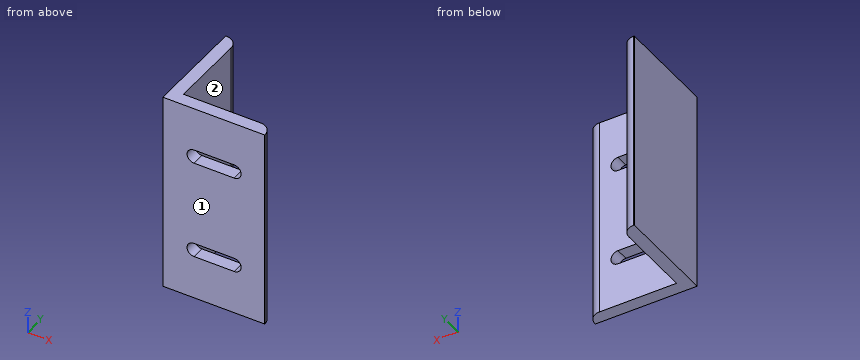
```python
from build123d import *

# Parameters (mm, degrees)
BOSS_EXTRUDE1_DEPTH = 100.4
CUT_EXTRUDE1_DEPTH  = 10


with BuildPart() as part:
    # Sketch1 → Boss-Extrude1 (new body)
    with BuildSketch(Plane.XY):
        with BuildLine():
            Line((44.8, 6.35), (12.35, 6.35))
            Line((12.35, 6.35), (6.35, 6.35))
            Line((6.35, 6.35), (6.35, 44.8))
            ThreePointArc((6.35, 44.8), (4.592640687, 49.042640687), (0.35, 50.8))
            Line((0.35, 50.8), (0, 50.8))
            Line((0, 50.8), (0, 6.35))
            Line((0, 6.35), (0, 0))
            Line((0, 0), (6.35, 0))
            Line((6.35, 0), (50.8, 0))
            Line((50.8, 0), (50.8, 0.35))
            ThreePointArc((50.8, 0.35), (49.042640687, 4.592640687), (44.8, 6.35))
        make_face()
    extrude(amount=BOSS_EXTRUDE1_DEPTH)

    # Sketch2 → Cut-Extrude1 (cut)
    with BuildSketch(Plane(origin=(0, 6.35, 0), x_dir=(1, 0, 0), z_dir=(0, 1, 0))):
        with BuildLine():
            Line((15.575, -21.9), (35.575, -21.9))
            ThreePointArc((35.575, -21.9), (39.075, -25.4), (35.575, -28.9))
            Line((35.575, -28.9), (15.575, -28.9))
            ThreePointArc((15.575, -28.9), (12.075, -25.4), (15.575, -21.9))
        make_face()
        with BuildLine():
            Line((15.575, -78.5), (35.575, -78.5))
            ThreePointArc((35.575, -78.5), (39.075, -75), (35.575, -71.5))
            Line((35.575, -71.5), (15.575, -71.5))
            ThreePointArc((15.575, -71.5), (12.075, -75), (15.575, -78.5))
        make_face()
    extrude(amount=-CUT_EXTRUDE1_DEPTH, mode=Mode.SUBTRACT)


solid = part.part
```
Build history of the part. All positions in model axes, mm. Face numbers are marked on the shaded views. A direction names the side the tool comes from. Round coordinates to 2 decimals unless told otherwise and drop trailing zeros. Write each loop counter-clockwise with the first axis right and the second up, starting at its lowest first coordinate (ties: lowest second). Pieces come first, ordered by that corner, then holes.
1) Pin check, flat tips, straight feed: pin 1 (1 mm diameter, centred on x = 25.5, z = 51, fed in from +Y); pin 2 (19 mm diameter, centred on y = 30.5, z = 72.5, fed in from +X). Stop position of each tip, or through.
2) Band-saw the part on A-A, the plane x = 24.5. List the corners of the cut face in (y, z), and give its area (3 significant figures).
3) Drill centre lines: probe 1 along Z at (x, y) = (37, 3); probe 2 along X at (y, z) = (35.5, 75). Where is each one in solid material? Low to high.
4) Band-saw the part on C-C, the plane z = 55. List the corners of the cut face in (x, y).
5) 3-axis set-ups, long thin cutter, end or side, ignore diameter. For the marked faces 1 and 2: which of +Z, -Z, +X, -X, +Y, -Y reach the whole face in a straight line?
6) Band-saw the part on B-B, the plane z = 75. List the corners of the cut face in (x, y) (3 decimals), and give its area (3 significant figures).
7) Band-saw the part on D-D, the plane y = 15.5. List the corners of the cut face in (x, z).
Ans:
1. pin 1: stops at y = 6.35
1. pin 2: stops at x = 6.35
2. outline: (0, 0) - (6.35, 0) - (6.35, 21.9) - (0, 21.9) - close; (0, 28.9) - (6.35, 28.9) - (6.35, 71.5) - (0, 71.5) - close; (0, 78.5) - (6.35, 78.5) - (6.35, 100.4) - (0, 100.4) - close
2. area: 549 mm2
3. probe 1: z = 0 to 22.2, 28.6 to 71.8, 78.2 to 100.4
3. probe 2: x = 0 to 6.35
4. outline: (0, 0) - (50.8, 0) - (50.8, 0.35) arc R6 ccw to (44.8, 6.35) - (6.35, 6.35) - (6.35, 44.8) arc R6 ccw to (0.35, 50.8) - (0, 50.8) - close
5. face 1: +Z, -Z, +X, -X, -Y
5. face 2: +Z, -Z, +X, +Y
6. outline: (0, 0) - (12.075, 0) - (12.075, 6.35) - (6.35, 6.35) - (6.35, 44.8) arc R6 ccw to (0.35, 50.8) - (0, 50.8) - close; (39.075, 0) - (50.8, 0) - (50.8, 0.35) arc R6 ccw to (44.8, 6.35) - (39.075, 6.35) - close
6. area: 418 mm2
7. outline: (0, 0) - (6.35, 0) - (6.35, 100.4) - (0, 100.4) - close
